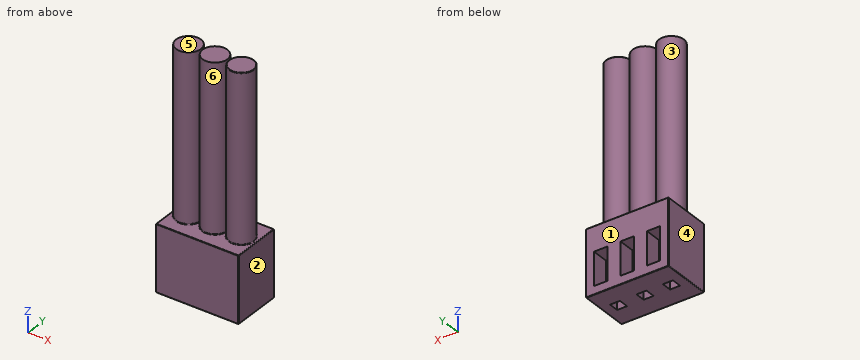
```python
from build123d import *

# Parameters (mm, degrees)
SKETCH_1_W          = 5
SKETCH_1_H          = 3
EXTRUDE_1_DEPTH     = 4
SKETCH_2_R          = 0.75
EXTRUDE_5_DEPTH     = 10
SKETCH_4_W          = 0.8
SKETCH_4_H          = 2
CUT_EXTRUDE_1_DEPTH = 1
SKETCH_5_W          = 0.6
SKETCH_5_H          = 0.6
CUT_EXTRUDE_2_DEPTH = 2
FILLET_1_R          = 0.04


with BuildPart() as part:
    # 草圖1 → 填料-伸長1 (new body)
    with BuildSketch(Plane.XY):
        with Locations((0.05874417, -0.145833333)):
            Rectangle(SKETCH_1_W, SKETCH_1_H)
    extrude(amount=EXTRUDE_1_DEPTH)

    # 草圖2 → 填料-伸長5 (add)
    with BuildSketch(Plane.XY.offset(4)):
        with Locations((-1.54125583, -0.145833333)):
            Circle(SKETCH_2_R)
        with Locations((0.05874417, -0.145833333)):
            Circle(SKETCH_2_R)
        with Locations((1.65874417, -0.145833333)):
            Circle(SKETCH_2_R)
    extrude(amount=EXTRUDE_5_DEPTH)

    # 草圖4 → 除料-伸長1 (cut)
    with BuildSketch(Plane(origin=(0, 1.354166667, 0), x_dir=(1, 0, 0), z_dir=(0, 1, 0))):
        with Locations((1.65874417, -1.5)):
            Rectangle(SKETCH_4_W, SKETCH_4_H)
        with Locations((0.05874417, -1.5)):
            Rectangle(SKETCH_4_W, SKETCH_4_H)
        with Locations((-1.54125583, -1.5)):
            Rectangle(SKETCH_4_W, SKETCH_4_H)
    extrude(amount=-CUT_EXTRUDE_1_DEPTH, mode=Mode.SUBTRACT)

    # 草圖5 → 除料-伸長2 (cut)
    with BuildSketch(Plane(origin=(0, 0, 0), x_dir=(-1, 0, 0), z_dir=(0, 0, -1))):
        with Locations((-1.65874417, -0.145833333)):
            Rectangle(SKETCH_5_W, SKETCH_5_H)
        with Locations((-0.05874417, -0.145833333)):
            Rectangle(SKETCH_5_W, SKETCH_5_H)
        with Locations((1.54125583, -0.145833333)):
            Rectangle(SKETCH_5_W, SKETCH_5_H)
    extrude(amount=-CUT_EXTRUDE_2_DEPTH, mode=Mode.SUBTRACT)

    # 圓角1
    fillet_1_edges = [part.edges().sort_by_distance(p)[0] for p in [
        (2.55874417, -0.145833333, 4),
        (0.05874417, 1.354166667, 4),
        (-2.29125583, -0.145833333, 4),
        (-0.69125583, -0.145833333, 4),
        (0.90874417, -0.145833333, 4),
        (0.90874417, -0.145833333, 14),
        (-2.44125583, -0.145833333, 4),
        (0.05874417, 1.354166667, 0),
        (2.55874417, -0.145833333, 0),
        (0.05874417, -1.645833333, 0),
        (-2.44125583, -0.145833333, 0),
        (0.05874417, -1.645833333, 4),
        (-2.44125583, 1.354166667, 2),
        (2.55874417, 1.354166667, 2),
        (2.55874417, -1.645833333, 2),
        (-2.44125583, -1.645833333, 2),
    ]]
    fillet(fillet_1_edges, radius=FILLET_1_R)


solid = part.part
```
CAD build for the part. Positions are in the model's coordinates, mm. Face numbers are marked on the shaded views. A direction names the side the tool comes from. Give positions to 0.01 mm unless a question says otherwise; leave off trailing zeros. Loops run counter-clockwise (first coordinate to the right, second up) from the corner with the lowest first, then second, coordinate; pieces in that order, holes last. Notation, with made-up numbers: M 23.25,57 L 28.25,57 A13 cw 28.25,64 Z; hole C -9,63.25 d3. An arc over 180 degrees is marked long. Use one line per item in the form item = value.
Item 1: Slice it at A-A (y = 1). List the corners of the cut face in (x, z), plus the area to 3 significant figures.
Determined:
outline = M -2.44,0.04 A0.04 ccw -2.4,0 L 2.52,0 A0.04 ccw 2.56,0.04 L 2.56,3.96 A0.04 ccw 2.52,4 L -2.4,4 A0.04 ccw -2.44,3.96 Z; hole M -1.94,0.5 L -1.14,0.5 L -1.14,2.5 L -1.94,2.5 Z; hole M -0.34,0.5 L 0.46,0.5 L 0.46,2.5 L -0.34,2.5 Z; hole M 1.26,0.5 L 2.06,0.5 L 2.06,2.5 L 1.26,2.5 Z
area = 15.2 mm2
Item 2: Which spindle directions (+Z, -Z, +X, -X, +Y, -Y) get a long thin tool onto all of the face, cutting with end or side? Do the marked faces 5 and 6. Say none if no direction does.
Determined:
face_5 = +Z, +X, -X, +Y, -Y
face_6 = +Z
Item 3: Flat gauge pins, fed straight in: pin 1 (0.5 mm diameter, centred on x = 2, z = 1, fed in from +Y); pin 2 (3 mm diameter, centred on x = 1, z = 6, fed in from -Y). Where does each tip first touch, or does it go through?
Determined:
pin_1 = 1.35
pin_2 = -0.9
Item 4: Drill centre lines: probe 1 along Z at (x, y) = (-1.8, 1.1); probe 2 along Y at (x, z) = (0.3, 1); probe 3 along X at (y, z) = (-0.5, 7). Where is each one in solid material? Low to high. Write a range as from..to.
Determined:
probe_1 = 0..0.5, 2.5..4
probe_2 = -1.65..-0.45, 0.15..0.35
probe_3 = -2.2..-0.88, -0.6..0.72, 1..2.32
Item 5: Two-plate mould, pull along X, no slides. Class the marked faces 1, 2, 3 and 4: pulls with the +X half, pulls with the -X half, needs draft (parallel to the pull), parting line crosses it, or undercut.
Determined:
face_1 = needs draft
face_2 = pulls with the +X half
face_3 = undercut
face_4 = pulls with the -X half
Item 6: Slice it at B-B (y = -1.4). List the corners of the cut face in (x, z).
Determined:
outline = M -2.44,0.04 A0.04 ccw -2.4,0 L 2.52,0 A0.04 ccw 2.56,0.04 L 2.56,3.96 A0.04 ccw 2.52,4 L -2.4,4 A0.04 ccw -2.44,3.96 Z
Item 7: Slice it at C-C (z = 12.5). List the corners of the cut face in (x, y).
Determined:
outline = C -1.54,-0.15 d1.5; C 0.06,-0.15 d1.5; C 1.66,-0.15 d1.5
